Here's how the part is built. I have some questions about the finished solid (model axes, mm). Face numbers are marked on the shaded views. Give positions to 0.01 mm unless a question says otherwise; leave off trailing zeros. Loops run counter-clockwise (first coordinate to the right, second up) from the corner with the lowest first, then second, coordinate; pieces in that order, holes last. Notation, with made-up numbers: M 39,-15.75 L 75,-15.75 A32 ccw 75,18.25 Z; hole C 69.5,8 d8. An arc over 180 degrees is marked long. Write item = value, one per line. Start each with the question number.
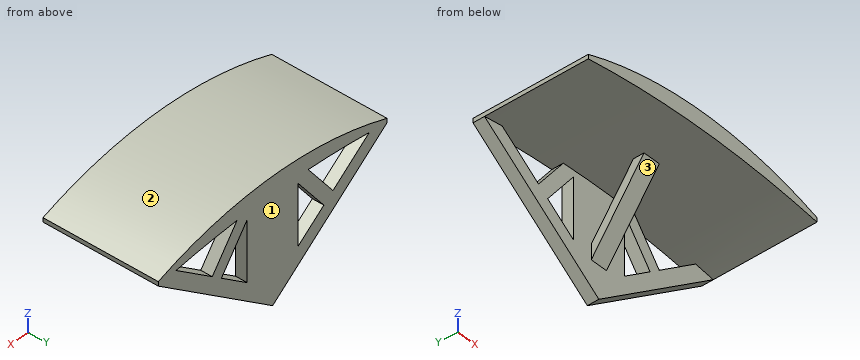
Autodesk Fusion 360 part; units mm, degrees
sketch "Sketch1" plane through (0, 0, 0) normal (0, 1, 0) x (1, 0, 0)
  line L0 (0, 0) -> (-90, 0)
  line L1 (-90, 0) -> (-90, -8)
  line L2 (-90, -8) -> (0, -8)
  line L3 (0, -8) -> (0, 0)
  arc A0 (-90, 0) -> (0, 0) centre (-45, 122.5625) ccw
  line L4 (-90, 0) -> (0, 0)
  line L5 (0, 0) -> (0, 1.5)
  line L6 (0, 1.5) -> (-90, 1.5)
  line L7 (-90, 1.5) -> (-90, 0)
  arc A1 (-90, 1.5) -> (0, 1.5) centre (-45, 287.9873) ccw
  dimension "d1" = 8
  dimension "d2" = 90
  dimension "d3" = 1.5
  dimension "d4" = 290
extrude "Extrude1" add sketch "Sketch1" along normal blind 40 contours L0 A0 L4 A1 | L0 L4 L5 A1 | L0 L4 L7 A1
sketch "Sketch2" plane through (0, 40, 0) normal (0, 1, 0) x (-1, 0, 0)
  arc A0 (90, 0) -> (0, 0) centre (45, -122.5625) ccw
  line L0 (0, 0) -> (0, -1.5)
  arc A1 (90, -1.5) -> (0, -1.5) centre (45, -287.9873) ccw
  line L1 (90, -1.5) -> (90, 0)
  line L2 (90, -1.5) -> (45, -35.4099)
  line L3 (45, -35.4099) -> (0, -1.5)
  line L4 (83.0298, -0.4917) -> (45, -29.1493)
  line L5 (45, -29.1493) -> (6.9702, -0.4917)
  line L6 (45, -35.4099) -> (45, 3)
  line L7 (55, -21.6137) -> (55, 1.8402)
  line L8 (55, 1.8402) -> (45, 3)
  line L9 (45, 3) -> (35, 1.8402)
  line L10 (59.0023, 1.6744) -> (68.7457, -11.2556)
  line L11 (6.9702, -0.4917) -> (83.0298, -0.4917)
  line L12 (55, -0.4917) -> (65.1519, -13.9637)
  line L13 (30.9977, 1.6744) -> (21.2543, -11.2556)
  line L14 (35, -0.4917) -> (24.8481, -13.9637)
  line L15 (35, -21.6137) -> (35, 1.8402)
  dimension "d8" = 10
  dimension "d9" = 5
  dimension "d10" = 5
  dimension "d13" = 37
  dimension "d14" = 90
  dimension "d15" = 4.5
extrude "Extrude2" add sketch "Sketch2" against normal blind 4 contours A1 L2 L4 L6 | A1 L3 L5 L6 | A1 L7 L10 L11 | L4 L10 L11 L12 | L4 L6 L7 L11 | L5 L6 L11 L15 | A1 L11 L13 L15 | L5 L11 L13 L14 | A1 L6 L7 L11 | A1 L6 L11 L15
ref_plane "WorkPlane1" through (-45, 0, 0) normal (1, 0, 0) x (0, 1, 0)
sketch "Sketch3" plane through (-45, 0, 0) normal (1, 0, 0) x (0, 1, 0)
  line L0 (17, 3) -> (36, -24)
  line L1 (36, -24) -> (36, -18.7871)
  line L2 (36, -18.7871) -> (20.2674, 3.5698)
  line L3 (20.2674, 3.5698) -> (17, 3)
  dimension "d17" = 3
extrude "Extrude3" add sketch "Sketch3" along normal mid plane 6
Q1. Will these pins go through, and if not, where does the flat tip stop? pin 1 (12 mm diameter, centred on x = -15, z = -20, fed in from -Y); pin 2 (8 mm diameter, centred on x = -33.5, z = -28, fed in from +Y); pin 3 (3 mm diameter, centred on y = 38, z = -14.5, fed in from -X); pin 4 (3 mm diameter, centred on y = 37.5, z = -14.5, fed in from +X).
Q2. If we section it at B-B, the plane y = 25: List the corners of the cut face in (x, z) for me (1 decimal).
Q3. If we section it at C-C, the plane z = -12.5: List the corners of the cut face in (x, y) for me.
Q4. If I drill on line 1 along Y through (x, z) = (-78.5, -8); line 2 along X through (y, z) = (32, -17.5); line 3 along Z through (x, y) = (-77, 12.5), over which ranges is the centre line in solid material (lowest first)?
Q5. If we section it at D-D, the plane x = -72: List the corners of the cut face in (y, z) for me, then the cut area to 3 significant figures.
Q6. If we section it at A-A, the plane z = -2.5: List the corners of the cut face in (x, y) for me, then the cut area to 3 significant figures.
Q7. We'd pull the mould along Y, two halves only. Please class the marked faces 1, 2 and 3: pulls with the +Y half, pulls with the -Y half, needs draft (parallel to the pull), parting line crosses it, or undercut.
Resolved:
q1.pin_1 = 36
q1.pin_2 = 40
q1.pin_3 = -74.74
q1.pin_4 = -15.26
q2.outline = M -90,-1.5 A290 cw 0,-1.5 L 0,0 A130.6 ccw -90,0 Z; M -48,-8.4 L -42,-8.4 L -42,-3.2 L -48,-3.2 Z
q3.outline = M -75.4,36 L -64.05,36 L -64.05,40 L -75.4,40 Z; M -55,36 L -35,36 L -35,40 L -55,40 Z; M -48,27.91 L -42,27.91 L -42,31.58 L -48,31.58 Z; M -25.95,36 L -14.6,36 L -14.6,40 L -25.95,40 Z
q4.line_1 = 36 to 40
q4.line_2 = -48 to -42
q4.line_3 = 0.24 to 4.02
q5.outline = M 0,0.75 L 40,0.75 L 40,5.18 L 0,5.18 Z; M 36,-15.06 L 40,-15.06 L 40,-8.8 L 36,-8.8 Z
q5.area = 202 mm²
q6.outline = M -88.67,36 L -80.36,36 L -80.36,40 L -88.67,40 Z; M -62.15,36 L -56.51,36 L -56.51,40 L -62.15,40 Z; M -55,36 L -35,36 L -35,40 L -55,40 Z; M -48,20.87 L -42,20.87 L -42,24.54 L -48,24.54 Z; M -33.49,36 L -27.85,36 L -27.85,40 L -33.49,40 Z; M -9.64,36 L -1.33,36 L -1.33,40 L -9.64,40 Z
q6.area = 214 mm²
q7.face_1 = pulls with the +Y half
q7.face_2 = needs draft
q7.face_3 = pulls with the -Y half
